```python
from build123d import *

# Parameters (mm, degrees)
SKETCH1_W           = 70
SKETCH1_H           = 55
SKETCH1_R           = 16
BOSS_EXTRUDE1_DEPTH = 5
SKETCH2_R           = 3
CUT_EXTRUDE1_DEPTH  = 45.791182168
FILLET1_R           = 10


with BuildPart() as part:
    # Sketch1 → Boss-Extrude1 (new body)
    with BuildSketch(Plane(origin=(0, 0, 0), x_dir=(1, 0, 0), z_dir=(0, 1, 0))):
        Rectangle(SKETCH1_W, SKETCH1_H)
        with Locations(Location((0, 10, 0), (0, 0, 270))):
            Circle(SKETCH1_R, mode=Mode.SUBTRACT)
    extrude(amount=BOSS_EXTRUDE1_DEPTH)

    # Sketch2 → Cut-Extrude1 (cut, through all)
    with BuildSketch(Plane(origin=(0, 5, 0), x_dir=(1, 0, 0), z_dir=(0, 1, 0))):
        with Locations(Location((-17.5, -20.310889132, 0), (0, 0, 270))):
            Circle(SKETCH2_R)
        with Locations(Location((17.5, -20.310889132, 0), (0, 0, 270))):
            Circle(SKETCH2_R)
    extrude(amount=-CUT_EXTRUDE1_DEPTH, mode=Mode.SUBTRACT)

    # Fillet1
    fillet1_edges = [part.edges().sort_by_distance(p)[0] for p in [
        (35, 2.5, -27.5),
    ]]
    fillet(fillet1_edges, radius=FILLET1_R)


solid = part.part
```
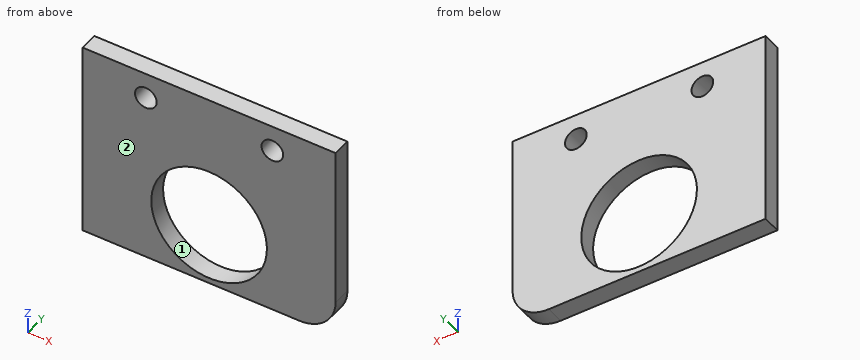
The listing builds one solid part. Answer for the finished solid, in the listing's coordinates (mm). Face numbers are marked on the shaded views. Give positions to 0.01 mm unless a question says otherwise; leave off trailing zeros. Write each loop counter-clockwise with the first axis right and the second up, starting at its lowest first coordinate (ties: lowest second). Pieces come first, ordered by that corner, then holes. Notation, with made-up numbers: (9, 29.25) -> (31, 29.25) arc R26 ccw to (31, 54.25) -> close; hole circle Ø9 at (12.25, 27). An arc over 180 degrees is marked (long way). Use one line per item in the form item = value.
1) For a pull along X with two mould halves and no side action, classify the marked faces 1 and 2 as +X half, -X half, draft (parallel to the pull), parting line (faces both ways), or undercut.
Result:
face_1 = undercut
face_2 = draft
2) Section C-C on y = 2.25 is taken. Write down the section's boundary in (x, z), plus the area to 3 significant figures.
Result:
outline = (-35, -27.5) -> (25, -27.5) arc R10 ccw to (35, -17.5) -> (35, 27.5) -> (-35, 27.5) -> close; hole circle Ø6 at (-17.5, 20.31); hole circle Ø32 at (0, -10); hole circle Ø6 at (17.5, 20.31)
area = 2,970 mm²
3) Section A-A on z = 0 is taken. Write down the section's boundary in (x, y), plus the area to 3 significant figures.
Result:
outline = (-35, 0) -> (-12.49, 0) -> (-12.49, 5) -> (-35, 5) -> close; (12.49, 0) -> (35, 0) -> (35, 5) -> (12.49, 5) -> close
area = 225 mm²
4) Section D-D on z = 20 is taken. Write down the section's boundary in (x, y), plus the area to 3 significant figures.
Result:
outline = (-35, 0) -> (-20.48, 0) -> (-20.48, 5) -> (-35, 5) -> close; (-14.52, 0) -> (14.52, 0) -> (14.52, 5) -> (-14.52, 5) -> close; (20.48, 0) -> (35, 0) -> (35, 5) -> (20.48, 5) -> close
area = 290 mm²
5) Section B-B on x = 0 is taken. Write down the section's boundary in (y, z).
Result:
outline = (0, -27.5) -> (5, -27.5) -> (5, -26) -> (0, -26) -> close; (0, 6) -> (5, 6) -> (5, 27.5) -> (0, 27.5) -> close
6) This flat-tipped pin is pushed along its axis until it touches: P1, Ø1.5, axis at x = -26.5, z = 19.5, coming from the -Y side. Where does it stop, or does it pass through?
Result:
P1 = 0
7) Straight lines are drawn through the part: probe 1 along X at (y, z) = (0.75, 20); probe 2 along X at (y, z) = (3.1, -10); probe 3 along X at (y, z) = (4.3, 21). For each, find the intervals that lie inside material, in ascending order.
Result:
probe_1 = -35 to -20.48, -14.52 to 14.52, 20.48 to 35
probe_2 = -35 to -16, 16 to 35
probe_3 = -35 to -20.42, -14.58 to 14.58, 20.42 to 35
